```python
from build123d import *

# Parameters (mm, degrees)
SKETCH1_W                                      = 210
SKETCH1_H                                      = 30
EXTRUDE1_DEPTH                                 = 20
CBORE_FOR_M6_HEX_HEAD_FLANGE_BOLT1_D           = 6.6
CBORE_FOR_M6_HEX_HEAD_FLANGE_BOLT1_CBORE_D     = 16
CBORE_FOR_M6_HEX_HEAD_FLANGE_BOLT1_CBORE_DEPTH = 6.6
CUT_EXTRUDE1_REACH                             = 32
SKETCH4_W                                      = 80
SKETCH4_H                                      = 0.5
M6_TAPPED_HOLE1_D                              = 5


with BuildPart() as part:
    # Sketch1 → Extrude1 (new body)
    with BuildSketch(Plane.XY):
        Rectangle(SKETCH1_W, SKETCH1_H)
    extrude(amount=EXTRUDE1_DEPTH)

    # CBORE for M6 Hex Head Flange Bolt1 (through all)
    with Locations(Plane(origin=(0, 0, 0), x_dir=(-1, 0, 0), z_dir=(0, 0, -1))):
        with Locations((82.5, 0), (-82.5, 0)):
            CounterBoreHole(CBORE_FOR_M6_HEX_HEAD_FLANGE_BOLT1_D / 2, CBORE_FOR_M6_HEX_HEAD_FLANGE_BOLT1_CBORE_D / 2, CBORE_FOR_M6_HEX_HEAD_FLANGE_BOLT1_CBORE_DEPTH)

    # Sketch4 → Cut-Extrude1 (cut, up to next)
    with BuildSketch(Plane(origin=(0, 15, 0), x_dir=(1, 0, 0), z_dir=(0, 1, 0)), mode=Mode.PRIVATE) as cut_extrude1_sk1:
        with Locations((0, -19.75)):
            Rectangle(SKETCH4_W, SKETCH4_H)
    cut_extrude1_tool1 = extrude(cut_extrude1_sk1.sketch, amount=-CUT_EXTRUDE1_REACH, mode=Mode.PRIVATE) & part.part
    add(cut_extrude1_tool1.solids().sort_by_distance((0, 15, 19.75))[0], mode=Mode.SUBTRACT)

    # M6 Tapped Hole1 (through all)
    with Locations(Plane.XY.offset(19.5)):
        with Locations((-23, 0), (23, 0)):
            Hole(M6_TAPPED_HOLE1_D / 2)


solid = part.part
```
CAD build for the part. Positions are in the model's coordinates, mm. A direction names the side the tool comes from. Round coordinates to 2 decimals unless told otherwise and drop trailing zeros. Write each loop counter-clockwise with the first axis right and the second up, starting at its lowest first coordinate (ties: lowest second). Pieces come first, ordered by that corner, then holes. Notation, with made-up numbers: (61, 50.25) -> (118, 50.25) arc R25 ccw to (118, 63.25) -> close; hole circle Ø2 at (87.25, -4.75). An arc over 180 degrees is marked (long way). Answer in a Markdown table with one row per item. Add a question column.
Item 1: Mould opens along X. For faces 1 (the face through (72, 0, 20)), 2 (the face through (-76.151, -4.868, 3.254)), 3 (the face through (-105, 0, 10)) say: pulls with the +X half, pulls with the -X half, needs draft (parallel to the pull), parting line crosses it, or undercut.
Item 2: Saw through at B-B, the plane z = 9. Write the cut outline in (x, y), then the cut area to 3 significant figures.
Item 3: Drop flat-ended pins along their axis: pin 1 Ø3 at (x, y) = (-23, 0) entering from +Z; pin 2 Ø9 at (x, y) = (-9.5, 0.5) entering from +Z; pin 3 Ø12 at (x, y) = (-22, 3.5) entering from -Z; pin 4 Ø10.5 at (x, y) = (82.5, 0) entering from -Z. Give the stop position or say it passes through.
Item 4: Saw through at C-C, the plane x = 23. Write the cut outline in (y, z).
Item 5: Drill centre lines: line 1 (Y direction, x = -82.5, z = 3); line 2 (Y direction, x = -82.5, z = 13.25); line 3 (Z direction, x = 12.5, y = 14). Where is each one in solid material? Low to high. Write a range as from..to.
Item 6: Saw through at A-A, the plane x = 82.5. Write the cut outline in (y, z).
Item 7: Saw through at D-D, the plane x = -35.5. Write the cut outline in (y, z), then the cut area to 3 significant figures.
Item 8: Which spindle directions (+Z, -Z, +X, -X, +Y, -Y) get a long thin tool onto all of the face, cutting with end or side? Do faces 4 (the face through (88.849, -4.868, 3.254)), 5 (the face through (-1, 0, 0)), 6 (the face through (-1, 0, 19.5)). Say none if no direction does.
Findings below:
| question | item | result |
|---|---|---|
| 1 | face 1 | needs draft |
| 1 | face 2 | undercut |
| 1 | face 3 | pulls with the -X half |
| 2 | outline | (-105, -15) -> (105, -15) -> (105, 15) -> (-105, 15) -> close; hole circle Ø6.6 at (-82.5, 0); hole circle Ø5 at (-23, 0); hole circle Ø5 at (23, 0); hole circle Ø6.6 at (82.5, 0) |
| 2 | area | 6,190 mm^2 |
| 3 | pin 1 | passes through |
| 3 | pin 2 | stops at z = 19.5 |
| 3 | pin 3 | stops at z = 0 |
| 3 | pin 4 | stops at z = 6.6 |
| 4 | outline | (-15, 0) -> (-2.5, 0) -> (-2.5, 19.5) -> (-15, 19.5) -> close; (2.5, 0) -> (15, 0) -> (15, 19.5) -> (2.5, 19.5) -> close |
| 5 | line 1 | y = -15..-8, 8..15 |
| 5 | line 2 | y = -15..-3.3, 3.3..15 |
| 5 | line 3 | z = 0..19.5 |
| 6 | outline | (-15, 0) -> (-8, 0) -> (-8, 6.6) -> (-3.3, 6.6) -> (-3.3, 20) -> (-15, 20) -> close; (3.3, 6.6) -> (8, 6.6) -> (8, 0) -> (15, 0) -> (15, 20) -> (3.3, 20) -> close |
| 7 | outline | (-15, 0) -> (15, 0) -> (15, 19.5) -> (-15, 19.5) -> close |
| 7 | area | 585 mm^2 |
| 8 | face 4 | -Z |
| 8 | face 5 | -Z, +X, -X, +Y, -Y |
| 8 | face 6 | +Z, +Y, -Y |
